from build123d import *

# Parameters (mm, degrees)
MODEL_R             = 1.500000008
MODEL_R_2           = 1.499950004
MODEL_R_3           = 1.500050014
MODEL_R_4           = 1.500000002
BOSS_EXTRUDE1_DEPTH = 3


with BuildPart() as part:
    # Model → Boss-Extrude1 (new body)
    with BuildSketch(Plane.XY):
        with BuildLine():
            Line((41.133407433, 54.383216824), (41.133407433, 44.212078484))
            Line((41.133407433, 44.212078484), (41.133407433, 27.226016824))
            add(Edge.make_bspline(
                [(41.133407433, 27.226016824), (41.133407433, 26.430416824), (41.449407433, 25.667416824), (42.012007433, 25.104816824)],
                knots=[0, 0, 0, 0, 0.333333333, 0.333333333, 0.333333333, 0.333333333], degree=3))
            add(Edge.make_bspline(
                [(42.012007433, 25.104816824), (42.574607433, 24.542216824), (43.337707433, 24.226016824), (44.133407433, 24.226016824)],
                knots=[0.333333333, 0.333333333, 0.333333333, 0.333333333, 1, 1, 1, 1], degree=3))
            Line((44.133407433, 24.226016824), (62.133207433, 24.226016824))
            ThreePointArc((62.133207433, 24.226016824), (64.254457434, 25.104766823), (65.133207433, 27.226016824))
            Line((65.133207433, 27.226016824), (65.133207433, 44.226016824))
            Line((65.133207433, 44.226016824), (65.133207433, 54.397160398))
            ThreePointArc((65.133207433, 54.397160398), (64.34779637, 56.530036555), (62.292266716, 57.5))
            Line((62.292266716, 57.5), (59.346369656, 57.5))
            Line((59.346369656, 57.5), (47.346484736, 57.5))
            Line((47.346484736, 57.5), (43.843018497, 57.5))
            ThreePointArc((43.843018497, 57.5), (41.866482804, 56.482116631), (41.133407433, 54.383216824))
        make_face()
        with Locations((44.499899992, 27.500000005)):
            Circle(MODEL_R, mode=Mode.SUBTRACT)
        with Locations((61.499949997, 27.500049997)):
            Circle(MODEL_R_2, mode=Mode.SUBTRACT)
        Polygon((50.4999, 52.5), (50.4999, 54), (55.4999, 54), (55.4999, 52.5), (58.9999, 52.5), (58.9999, 47), (61.9999, 47), (61.9999, 35), (58.9999, 35), (58.9999, 29.5), (55.4999, 29.5), (55.4999, 28.0001), (50.4999, 28.0001), (50.4999, 29.5), (46.9999, 29.5), (46.9999, 35), (44.0001, 35), (44.0001, 47), (46.9999, 47), (46.9999, 52.5), align=None, mode=Mode.SUBTRACT)
        with Locations((44.499849987, 54.700050007)):
            Circle(MODEL_R_3, mode=Mode.SUBTRACT)
        with Locations((61.499900002, 54.700099998)):
            Circle(MODEL_R_4, mode=Mode.SUBTRACT)
    extrude(amount=BOSS_EXTRUDE1_DEPTH)


solid = part.part
Source: CAD feature listing. Evaluate the final solid. Frame: model axes, mm. A direction names the side the tool comes from. Round coordinates to 2 decimals unless told otherwise and drop trailing zeros. Loops run counter-clockwise (first coordinate to the right, second up) from the corner with the lowest first, then second, coordinate; pieces in that order, holes last. Notation, with made-up numbers: (62, -32.5) - (91, -32.5) arc R32 ccw to (91, -1.5) - close; hole circle Ø4 at (21.25, -32). An arc over 180 degrees is marked (long way). Write item = value, one per line. Start each with the question number.
Item 1: Section query A-A on x = 46.5. Output: boundary loops of the cut face in (y, z), plus the area to 3 significant figures.
Item 2: Material intervals for line 1 (Y direction, x = 59.5, z = 2.25); line 2 (Y direction, x = 53.5, z = 1.7); line 3 (X direction, y = 43, z = 2.4), sorted ascending.
Item 3: Section query C-C on z = 0.75. Count the separate pieces of the cut face and the enclosed holes in it, plus the area to 3 significant figures.
Item 4: Section query B-B on y = 30.5. Output: boundary loops of the cut face in (x, z).
Item 5: Mould query, pull axis X, two halves, no side actions, for faces 3 (the face through (65.133, 41, 1)), 4 (the face through (41.89, 56.51, 1.48)), 5 (the face through (61, 35, 1)). Classes: released by +X, released by -X, zero draft, split by the parting line, or undercut.
Item 6: Reachability of faces 1 (the face through (64.23, 25.08, 1.48)), 2 (the face through (59, 32, 1)) from +Z, -Z, +X, -X, +Y, -Y: full face, straight path, thin tool, end or side. Return the list, or none.
Item 7: First-contact query: pin 1 Ø1.5 at (y, z) = (35.5, 2) entering from -X; pin 2 Ø2.5 at (x, y) = (61.5, 54.7) entering from +Z. Flat tips, straight axial feed; report the tip coordinate or a pass-through.
Results list:
q1.outline = (24.23, 0) - (35, 0) - (35, 3) - (24.23, 3) - close; (47, 0) - (57.5, 0) - (57.5, 3) - (47, 3) - close
q1.area = 63.8 mm²
q2.line_1 = 24.23 to 35, 47 to 57.5
q2.line_2 = 24.23 to 28, 54 to 57.5
q2.line_3 = 41.13 to 44, 62 to 65.13
q3.separate_pieces = 1
q3.enclosed_holes = 5
q3.area = 400 mm²
q4.outline = (41.13, 0) - (47, 0) - (47, 3) - (41.13, 3) - close; (59, 0) - (65.13, 0) - (65.13, 3) - (59, 3) - close
q5.face_3 = released by +X
q5.face_4 = released by -X
q5.face_5 = undercut
q6.face_1 = +Z, -Z, +X, -Y
q6.face_2 = +Z, -Z
q7.pin_1 = 41.13
q7.pin_2 = through
